Input: part model. Units: mm. Frame: model coordinates. Face numbers are marked on the shaded views. A direction names the side the tool comes from. Give positions to 0.01 mm unless a question says otherwise; leave off trailing zeros. Order: outer loops, then holes, each group sorted by start corner. A loop starts at its lowest first (then second) coordinate and runs counter-clockwise, first axis right, second up. Notation, with made-up numbers: (-40, 32.25) - (16, 32.25) arc R25 ccw to (16, 65.25) - close; hole circle Ø3 at (-18.5, 45.5). An arc over 180 degrees is marked (long way). Answer in a Markdown table with one row per item. Add a question column.
1. Contact query for flat-ended pins moving along their axis: pin 1 (6.5 mm diameter, centred on x = 6.5, y = -13, fed in from +Z); pin 2 (9.5 mm diameter, centred on x = -2.68, z = 30, fed in from -Y); pin 3 (12 mm diameter, centred on y = -4, z = 0.5, fed in from +X); pin 4 (4 mm diameter, centred on x = 6, y = -17.5, fed in from +Z). Output: stop coordinate, or through.
2. Ray query, line 1 (Z direction, x = 0.75, y = -8.5); line 2 (X direction, y = -1.1, z = 30); line 3 (Z direction, x = 3.5, y = -11). Return the intervals inside material, ascending. Write a range as [from, to].
3. Mould query, pull axis Y, two halves, no side actions, for the marked faces 6, 7 and 8. Classes: released by +Y, released by -Y, zero draft, split by the parting line, or undercut.
4. Access query for the marked faces 1, 2, 3, 4 and 5. Directions: +Z, -Z, +X, -X, +Y, -Y. A direction counts if a zero-diameter tool reaches every point of the face in a straight line with its end or side. Return the directions, or none.
5. Section query B-B on z = 30. Return loops of the section in (x, y), and give its area (3 significant figures).
6. Section query C-C on y = -27. Return loops of the section in (x, z).
7. Section query D-D on z = 10.5. Return loops of the section in (x, y), and give its area (3 significant figures).
8. Section query A-A on x = 5. Return loops of the section in (y, z), and give its area (3 significant figures).
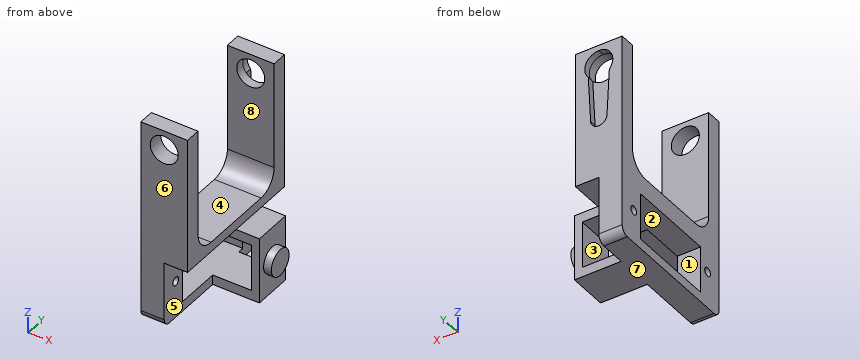
```python
from build123d import *
from build123d.topology import SkipClean

# Parameters (mm, degrees)
SKETCH2_W             = 12
SKETCH2_H             = 4
BOSS_EXTRUDE2_DEPTH   = 35
BOSS_EXTRUDE2_2_DEPTH = 35
SKETCH2_3_W           = 12
SKETCH2_3_H           = 29.15
BOSS_EXTRUDE3_DEPTH   = 2.5
SKETCH7_W             = 6
SKETCH7_H             = 37.15
BOSS_EXTRUDE4_DEPTH   = 17
CUT_EXTRUDE5_REACH    = 51.94
SKETCH8_R             = 1.1
SKETCH8_W             = 12
SKETCH8_H             = 23
CUT_EXTRUDE6_DEPTH    = 1.7
SKETCH10_R            = 3.6
CUT_EXTRUDE7_DEPTH    = 52.773465505
FILLET6_R             = 5
FILLET7_R             = 5
SKETCH12_W            = 2.5
SKETCH12_H            = 10
BOSS_EXTRUDE5_DEPTH   = 10
SKETCH13_W            = 17
SKETCH13_H            = 10
BOSS_EXTRUDE6_DEPTH   = 2
SKETCH14_R            = 3.4
BOSS_EXTRUDE7_DEPTH   = 2
FILLET8_R             = 2
FILLET9_R             = 2


with BuildPart() as part:
    # Sketch2 → Boss-Extrude2 (new body)
    with BuildSketch(Plane.XY):
        with Locations((-2.681545395, 0.036493048)):
            Rectangle(SKETCH2_W, SKETCH2_H)
    extrude(amount=BOSS_EXTRUDE2_DEPTH)

    # Sketch2_3 → Boss-Extrude3 (add)
    with BuildSketch(Plane.XY):
        with Locations((-2.681545395, -16.538506952)):
            Rectangle(SKETCH2_3_W, SKETCH2_3_H)
    extrude(amount=BOSS_EXTRUDE3_DEPTH)



with BuildPart() as body_2:
    # Sketch2 → Boss-Extrude2 2 (new body)
    with BuildSketch(Plane.XY):
        with Locations((-2.681545395, -33.113506952)):
            Rectangle(SKETCH2_W, SKETCH2_H)
    extrude(amount=BOSS_EXTRUDE2_2_DEPTH)


with BuildPart() as part_1:
    add(part.part)

    add(body_2.part)  # Boss-Extrude4 merges body 2
    # Sketch7 → Boss-Extrude4 (add)
    with BuildSketch(Plane(origin=(0, 0, 0), x_dir=(-1, 0, 0), z_dir=(0, 0, -1))):
        with Locations((5.681545395, -16.538506952)):
            Rectangle(SKETCH7_W, SKETCH7_H)
    extrude(amount=BOSS_EXTRUDE4_DEPTH)

    # Sketch8 → Cut-Extrude5 (cut, up to next)
    with BuildSketch(Plane(origin=(-2.681545395, 0, 0), x_dir=(0, 0, -1), z_dir=(1, 0, 0)), mode=Mode.PRIVATE) as cut_extrude5_sk1:
        with Locations((8.5, -2.388506952)):
            Circle(SKETCH8_R)
    cut_extrude5_tool1 = extrude(cut_extrude5_sk1.sketch, amount=-CUT_EXTRUDE5_REACH, mode=Mode.PRIVATE) & part_1.part
    # Sketch8 → Cut-Extrude5 (cut, up to next)
    with BuildSketch(Plane(origin=(-2.681545395, 0, 0), x_dir=(0, 0, -1), z_dir=(1, 0, 0)), mode=Mode.PRIVATE) as cut_extrude5_sk2:
        with Locations((7.5, -30.688506952)):
            Circle(SKETCH8_R)
    cut_extrude5_tool2 = extrude(cut_extrude5_sk2.sketch, amount=-CUT_EXTRUDE5_REACH, mode=Mode.PRIVATE) & part_1.part
    # Sketch8 → Cut-Extrude5 (cut, up to next)
    with BuildSketch(Plane(origin=(-2.681545395, 0, 0), x_dir=(0, 0, -1), z_dir=(1, 0, 0)), mode=Mode.PRIVATE) as cut_extrude5_sk3:
        with Locations((8.5, -16.538506952)):
            Rectangle(SKETCH8_W, SKETCH8_H)
    cut_extrude5_tool3 = extrude(cut_extrude5_sk3.sketch, amount=-CUT_EXTRUDE5_REACH, mode=Mode.PRIVATE) & part_1.part
    add(cut_extrude5_tool1.solids().sort_by_distance((-2.681545, -2.388507, -8.5))[0], mode=Mode.SUBTRACT)
    add(cut_extrude5_tool2.solids().sort_by_distance((-2.681545, -30.688507, -7.5))[0], mode=Mode.SUBTRACT)
    add(cut_extrude5_tool3.solids().sort_by_distance((-2.681545, -16.538507, -8.5))[0], mode=Mode.SUBTRACT)

    # Sketch9 → Cut-Extrude6 (cut)
    with BuildSketch(Plane(origin=(0, 2.036493048, 0), x_dir=(1, 0, 0), z_dir=(0, 1, 0))):
        with BuildLine():
            Line((-0.584210872, -15.668774056), (0.018454605, -27.61882382))
            ThreePointArc((0.018454605, -27.61882382), (-2.681545395, -33.6), (-5.381545395, -27.61882382))
            Line((-5.381545395, -27.61882382), (-4.778879917, -15.668774056))
            ThreePointArc((-4.778879917, -15.668774056), (-2.681545395, -13.674546931), (-0.584210872, -15.668774056))
        make_face()
    extrude(amount=-CUT_EXTRUDE6_DEPTH, mode=Mode.SUBTRACT)

    # Sketch10 → Cut-Extrude7 (cut, through all)
    with BuildSketch(Plane(origin=(0, 2.036493048, 0), x_dir=(1, 0, 0), z_dir=(0, 1, 0))):
        with Locations(Location((-2.681545395, -30, 0), (0, 0, 270))):
            Circle(SKETCH10_R)
    extrude(amount=-CUT_EXTRUDE7_DEPTH, mode=Mode.SUBTRACT)

    # Fillet6
    fillet6_edges = [part_1.edges().sort_by_distance(p)[0] for p in [
        (-2.681545395, -1.963506952, 2.5),
    ]]
    fillet(fillet6_edges, radius=FILLET6_R)

    # Fillet7
    fillet7_edges = [part_1.edges().sort_by_distance(p)[0] for p in [
        (-2.681545395, -31.113506952, 2.5),
    ]]
    fillet(fillet7_edges, radius=FILLET7_R)

    # Sketch12 → Boss-Extrude5 (add)
    with SkipClean():  # the faces are left unmerged after this step: merging them gives an invalid solid
        with BuildSketch(Plane(origin=(-2.681545395, 0, 0), x_dir=(0, 0, -1), z_dir=(1, 0, 0))):
            with Locations((1.25, -11.543506952)):
                Rectangle(SKETCH12_W, SKETCH12_H)
            with Locations((15.75, -11.543506952)):
                Rectangle(SKETCH12_W, SKETCH12_H)
        extrude(amount=BOSS_EXTRUDE5_DEPTH)

    # Sketch13 → Boss-Extrude6 (add)
    with SkipClean():  # the faces are left unmerged after this step: merging them gives an invalid solid
        with BuildSketch(Plane(origin=(7.318454605, 0, 0), x_dir=(0, 0, -1), z_dir=(1, 0, 0))):
            with Locations((8.5, -11.543506952)):
                Rectangle(SKETCH13_W, SKETCH13_H)
        extrude(amount=BOSS_EXTRUDE6_DEPTH)

    # Sketch14 → Boss-Extrude7 (add)
    with SkipClean():  # the faces are left unmerged after this step: merging them gives an invalid solid
        with BuildSketch(Plane(origin=(9.318454605, 0, 0), x_dir=(0, 0, -1), z_dir=(1, 0, 0))):
            with Locations(Location((8.5, -11.543506952, 0), (0, 0, 90))):
                Circle(SKETCH14_R)
        extrude(amount=BOSS_EXTRUDE7_DEPTH)

    # Fillet8
    fillet8_edges = [part_1.edges().sort_by_distance(p)[0] for p in [
        (-5.681545395, 2.036493048, -17),
    ]]
    fillet(fillet8_edges, radius=FILLET8_R)

    # Fillet9
    fillet9_edges = [part_1.edges().sort_by_distance(p)[0] for p in [
        (-5.681545395, -35.113506952, -17),
    ]]
    fillet(fillet9_edges, radius=FILLET9_R)


solid = part_1.part
```
Answer:
| question | item | result |
|---|---|---|
| 1 | pin 1 | stops at z = 2.5 |
| 1 | pin 2 | stops at y = -35.11 |
| 1 | pin 3 | stops at x = 9.32 |
| 1 | pin 4 | stops at z = 0 |
| 2 | line 1 | z = [-17, -14.5], [-2.5, 2.5] |
| 2 | line 2 | x = [-8.68, -6.28], [0.92, 3.32] |
| 2 | line 3 | z = [-17, -14.5], [-2.5, 0] |
| 3 | face 6 | released by -Y |
| 3 | face 7 | zero draft |
| 3 | face 8 | undercut |
| 4 | face 1 | +X, -X |
| 4 | face 2 | -X |
| 4 | face 3 | -X, +Y, -Y |
| 4 | face 4 | +Z, +X, -X |
| 4 | face 5 | -Z, +X, -Y |
| 5 | outline | (-8.68, -35.11) - (-6.28, -35.11) - (-6.28, -31.11) - (-8.68, -31.11) - close; (-8.68, -1.96) - (-6.28, -1.96) - (-6.28, 2.04) - (-8.68, 2.04) - close; (0.92, -35.11) - (3.32, -35.11) - (3.32, -31.11) - (0.92, -31.11) - close; (0.92, -1.96) - (3.32, -1.96) - (3.32, 2.04) - (0.92, 2.04) - close |
| 5 | area | 38.4 mm² |
| 6 | outline | (-8.68, -17) - (-2.68, -17) - (-2.68, -14.5) - (-8.68, -14.5) - close; (-8.68, -2.5) - (-2.68, -2.5) - (-2.68, 0) - (3.32, 0) - (3.32, 2.58) - (-8.68, 2.58) - close |
| 7 | outline | (-8.68, -35.11) - (3.32, -35.11) - (3.32, -31.11) - (-8.68, -31.11) - close; (-8.68, -1.96) - (3.32, -1.96) - (3.32, 2.04) - (-8.68, 2.04) - close |
| 7 | area | 96.0 mm² |
| 8 | outline | (-16.54, -17) - (-6.54, -17) - (-6.54, -14.5) - (-16.54, -14.5) - close; (-16.54, -2.5) - (-6.54, -2.5) - (-6.54, 0) - (-16.54, 0) - close |
| 8 | area | 50.0 mm² |
